Here's the drawing with two shaded views (mm, measured from the low corner). I have some questions. A direction names the side the tool comes from. Give positions to 0.01 mm unless a question says otherwise; leave off trailing zeros. Loops run counter-clockwise (first coordinate to the right, second up) from the corner with the lowest first, then second, coordinate; pieces in that order, holes last. Notation, with made-up numbers: (79.5, -21.75) - (96.5, -21.75) arc R35 cw to (96.5, 14.25) - close; hole circle Ø2 at (10.5, 44.25). An arc over 180 degrees is marked (long way). Use one line per item in the form item = value.
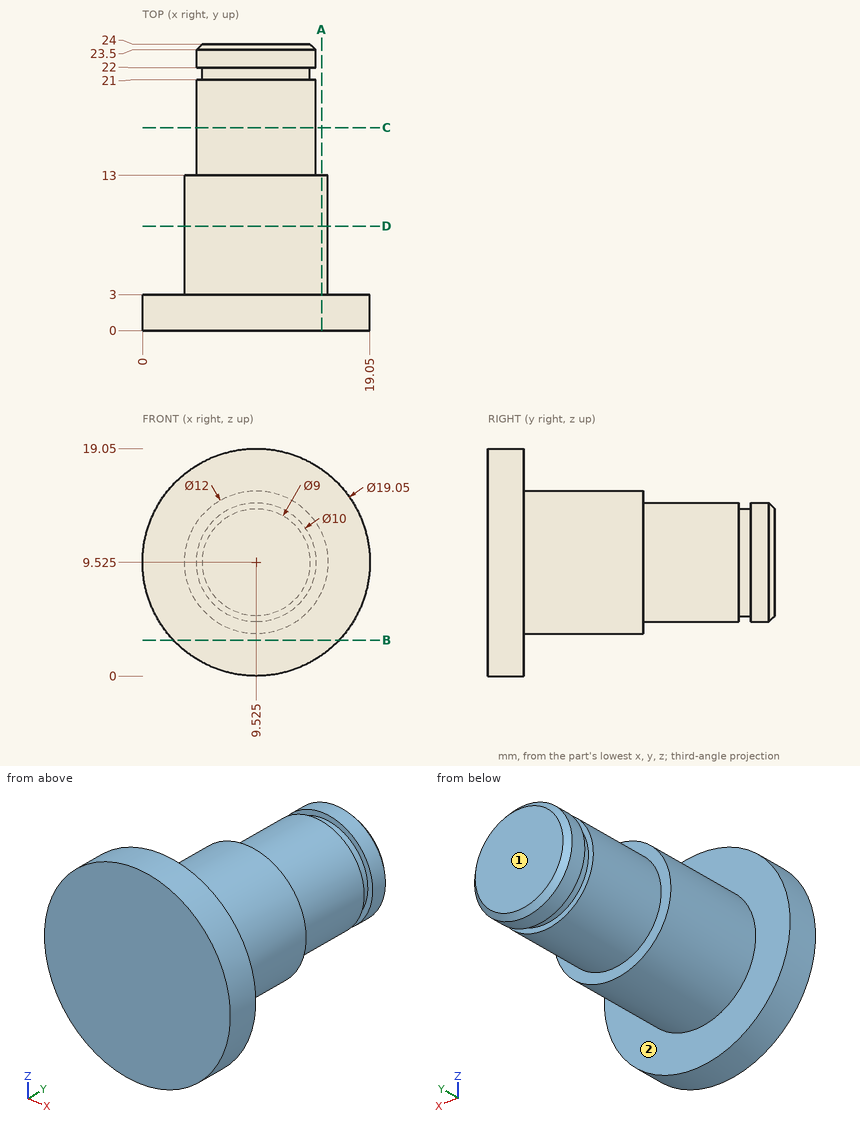
(1) If I drill on probe 1 along X at (y, z) = (2, 9.5); probe 2 along Z at (x, y) = (9.5, 10.75); probe 3 along Y at (x, z) = (7.25, 3.25), over which ranges is the centre line in solid material (lowest first)?
Geometry says:
probe_1 = 0 to 19.05
probe_2 = 3.53 to 15.52
probe_3 = 0 to 3
(2) For the marked faces 1 and 2, which set-ups out of +Z, -Z, +X, -X, +Y, -Y let a thin tool reach every point of the face, with its end or its side?
Geometry says:
face_1 = +Z, -Z, +X, -X, +Y
face_2 = +Y
(3) If we section it at B-B (z = 3): List the corners of the cut face in (x, y) for me.
Geometry says:
outline = (2.59, 0) - (16.46, 0) - (16.46, 3) - (2.59, 3) - close
(4) If we section it at C-C (y = 17): List the corners of the cut face in (x, z) for me (3 decimals), plus the area to 3 significant figures.
Geometry says:
outline = circle Ø10 at (9.525, 9.525)
area = 78.5 mm²
(5) If we section it at D-D (y = 8.75): List the corners of the cut face in (x, z) for me (3 decimals).
Geometry says:
outline = circle Ø12 at (9.525, 9.525)
(6) For P1, Ø10, axis at x = 4, y = 6.5, coming from the +Z side; P2, Ø3, axis at x = 10, y = 18, coming from the +Z side (3 decimals); P3, Ø1.5, axis at y = 16, z = 13.5, coming from the -X side, each with a flat end and sliding along its axis, tell me the tip position at first contact or that it passes through.
Geometry says:
P1 = 18.85
P2 = 14.525
P3 = 5.7
(7) If we section it at A-A (x = 15): List the corners of the cut face in (y, z) for me, plus the area to 3 significant figures.
Geometry says:
outline = (0, 1.73) - (3, 1.73) - (3, 7.07) - (13, 7.07) - (13, 11.98) - (3, 11.98) - (3, 17.32) - (0, 17.32) - close
area = 95.9 mm²
